from build123d import *

# Parameters (mm, degrees)
F0_R        = 10
F1_DEPTH    = 3
F2_R        = 2.95
F3_DEPTH    = 3.61
F4_R        = 3.05
F4_R_2      = 2.95
F5_DEPTH    = 5.23
F6_SIZE     = 1
F7_SIZE     = 0.5
F8_S5_R     = 2.95
F8_T6_DEPTH = 6


# Not quite as in the source:
# - a fillet or chamfer that OpenCascade refuses, or shapes differently, is made with other operations: its cross-section is extruded or revolved along the edge and cut away or added


with BuildPart() as f1:
    # F0 (on Top) → F1 (new body)
    with BuildSketch(Plane.XY):
        Circle(F0_R)
    extrude(amount=F1_DEPTH)

    # F2 (on face) → F3 (join)
    with BuildSketch(Plane.XY.offset(3)):
        Circle(F2_R)
    extrude(amount=F3_DEPTH)

    # F4 (on face) → F5 (join)
    with BuildSketch(Plane.XY.offset(6.61)):
        Circle(F4_R)
        Circle(F4_R_2, mode=Mode.SUBTRACT)
        Circle(F4_R_2)
    extrude(amount=F5_DEPTH)

    # F6
    f6_edges = [f1.edges().sort_by_distance(p)[0] for p in [
        (-3.05, 0, 11.84),
    ]]
    chamfer(f6_edges, length=F6_SIZE)

    # F7
    f7_edges = [f1.edges().sort_by_distance(p)[0] for p in [
        (-10, 0, 3),
        (-10, 0, 0),
    ]]
    chamfer(f7_edges, length=F7_SIZE)

    # F8: chamfer of 0.5 on 1 edges, made by hand


with BuildPart() as f8_tool2:
    # F8_s3 → F8_t4 (revolve)
    with BuildSketch(Plane.XZ):
        Polygon((2.55, 6.61), (3.05, 7.11), (3.05, 6.61), align=None)
    revolve(axis=Axis((0, 0, 6.61), (0, 0, 1)))

    # F8_s5 → F8_t6 (cut, symmetric)
    with BuildSketch(Plane.XY.offset(6.9)):
        Circle(F8_S5_R)
    extrude(amount=F8_T6_DEPTH, both=True, mode=Mode.SUBTRACT)


with BuildPart() as f1_1:
    add(f1.part)

    # F8_t1: cut F8_tool2
    add(f8_tool2.part, mode=Mode.SUBTRACT)


solid = f1_1.part
CAD build for the part. Positions are in the model's coordinates, mm. A direction names the side the tool comes from. Give positions to 0.01 mm unless a question says otherwise; leave off trailing zeros. Loops run counter-clockwise (first coordinate to the right, second up) from the corner with the lowest first, then second, coordinate; pieces in that order, holes last. Notation, with made-up numbers: M 22.25,-5 L 68.25,-5 A18 ccw 68.25,30 Z; hole C 82,14 d8. An arc over 180 degrees is marked long. Answer in a Markdown table with one row per item. Add a question column.
Item 1: Band-saw the part on D-D on z = 4. Give the cut face in (x, y), then the cut area to 3 significant figures.
Item 2: Tool access for faces 1 (the face through (-0.64, -2.88, 4.98)), 2 (the face through (-3.047, 0.134, 8.949)), 3 (the face through (0, 0, 11.84)): list every direction of +Z, -Z, +X, -X, +Y, -Y with a clear straight run to the whole face (end or side of a thin tool).
Item 3: Probe probe 1 along Z at (x, y) = (8, -1.5); probe 2 along X at (y, z) = (-3.75, 1.75); probe 3 along X at (y, z) = (3.5, 1.5). List the from-to ranges inside material, lowest first.
Item 4: Band-saw the part on C-C on z = 9.5. Give the cut face in (x, y), then the cut area to 3 significant figures.
Item 5: Drop flat-ended pins along their axis: P1, Ø2, axis at x = 4, z = 5.5, coming from the -Y side; P2, Ø1, axis at y = 3, z = 3, coming from the -X side; P3, Ø1.5, axis at x = -2.5, z = 4, coming from the -Y side; P4, Ø5, axis at x = 0, y = -6.5, coming from the +Z side. Give the stop position or say it passes through.
Item 6: Band-saw the part on A-A on y = 0. Give the cut face in (x, z), then the cut area to 3 significant figures.
Reply:
| question | item | result |
|---|---|---|
| 1 | outline | C 0,0 d5.9 |
| 1 | area | 27.3 mm^2 |
| 2 | face 1 | none |
| 2 | face 2 | +Z |
| 2 | face 3 | +Z, +X, -X, +Y, -Y |
| 3 | probe 1 | z = 0 to 3 |
| 3 | probe 2 | x = -9.27 to 9.27 |
| 3 | probe 3 | x = -9.37 to 9.37 |
| 4 | outline | C 0,0 d6.1 |
| 4 | area | 29.2 mm^2 |
| 5 | P1 | passes through |
| 5 | P2 | stops at x = -9.56 |
| 5 | P3 | stops at y = -2.37 |
| 5 | P4 | stops at z = 3 |
| 6 | outline | M -10,0.5 L -9.5,0 L 9.5,0 L 10,0.5 L 10,2.5 L 9.5,3 L 2.95,3 L 2.95,7.01 L 3.05,7.11 L 3.05,10.84 L 2.05,11.84 L -2.05,11.84 L -3.05,10.84 L -3.05,7.11 L -2.95,7.01 L -2.95,3 L -9.5,3 L -10,2.5 Z |
| 6 | area | 112 mm^2 |
